For this review, take the finished solid that the model builds, in its own axes (mm). Give positions to 0.01 mm unless a question says otherwise; leave off trailing zeros. Order: outer loops, then holes, each group sorted by start corner. A loop starts at its lowest first (then second) coordinate and runs counter-clockwise, first axis right, second up. Notation, with made-up numbers: M 78,68 L 126,68 A21 cw 126,93 Z; hole C -19.75,10.5 d10. An arc over 180 degrees is marked long. Answer as CSV lines item,"result". Start each with the question number.
1. We need section B-B, the plane x = -94.5. Give the boundary of the cut face in (y, z).
2. For line 1 along X through (y, z) = (7.5, 1.95); line 2 along Y through (x, z) = (106, 0.7), list the stretches that pass through material, from the lowest coordinate up.
3. We need section C-C, the plane z = 1.6. State how many separate pieces and enclosed holes the cut face has, and give its area (3 significant figures).
4. Clearance check with flat-ended pins moving along their axes: P1, Ø1.5, axis at y = -49, z = 2, coming from the -X side; P2, Ø1.5, axis at y = -50, z = 2, coming from the +X side; P3, Ø1.5, axis at x = 43.5, z = 1.5, coming from the -Y side. State where each tip first meets the part, or that it passes through.
5. We need section A-A, the plane y = -37. Give the boundary of the cut face in (x, z).
from build123d import *

# Parameters (mm, degrees)
SKETCH1_W           = 3
SKETCH1_H           = 27
BOSS_EXTRUDE1_DEPTH = 3
SKETCH2_W           = 3
SKETCH2_H           = 27
CUT_EXTRUDE1_DEPTH  = 10
SKETCH3_W           = 27
SKETCH3_H           = 5
BOSS_EXTRUDE3_DEPTH = 3


with BuildPart() as part:
    # Sketch1 → Boss-Extrude1 (new body)
    with BuildSketch(Plane.XY):
        Polygon((-90, 52.5), (-90, 47.5), (-113, 47.5), (-113, 52.5), (-140, 52.5), (-140, 47.5), (-150, 47.5), (-150, -47.5), (150, -47.5), (150, 47.5), (137, 47.5), (137, 52.5), (110, 52.5), (110, 47.5), (87, 47.5), (87, 52.5), (60, 52.5), (60, 47.5), (37, 47.5), (37, 52.5), (10, 52.5), (10, 47.5), (-13, 47.5), (-13, 52.5), (-40, 52.5), (-40, 47.5), (-63, 47.5), (-63, 52.5), align=None)
        with Locations((-147.5, 30.102605219)):
            Rectangle(SKETCH1_W, SKETCH1_H, mode=Mode.SUBTRACT)
        with Locations((-147.5, -29.897394781)):
            Rectangle(SKETCH1_W, SKETCH1_H, mode=Mode.SUBTRACT)
        with Locations((-147.5, 0.102605219)):
            Rectangle(SKETCH1_W, SKETCH1_H, mode=Mode.SUBTRACT)
    extrude(amount=BOSS_EXTRUDE1_DEPTH)

    # Sketch2 → Cut-Extrude1 (cut)
    with BuildSketch(Plane.XY.offset(3)):
        with Locations((141.5, 30.1)):
            Rectangle(SKETCH2_W, SKETCH2_H)
        with Locations((141.5, 0.1)):
            Rectangle(SKETCH2_W, SKETCH2_H)
        with Locations((141.5, -29.9)):
            Rectangle(SKETCH2_W, SKETCH2_H)
    extrude(amount=-CUT_EXTRUDE1_DEPTH, mode=Mode.SUBTRACT)

    # Sketch3 → Boss-Extrude3 (add)
    with BuildSketch(Plane.XY.offset(3)):
        with Locations((-126.5, -50)):
            Rectangle(SKETCH3_W, SKETCH3_H)
        with Locations((-76.5, -50)):
            Rectangle(SKETCH3_W, SKETCH3_H)
        with Locations((-26.5, -50)):
            Rectangle(SKETCH3_W, SKETCH3_H)
        with Locations((23.5, -50)):
            Rectangle(SKETCH3_W, SKETCH3_H)
        with Locations((73.5, -50)):
            Rectangle(SKETCH3_W, SKETCH3_H)
        with Locations((123.5, -50)):
            Rectangle(SKETCH3_W, SKETCH3_H)
    extrude(amount=-BOSS_EXTRUDE3_DEPTH)


solid = part.part
Result set:
1,outline,"M -47.5,0 L 47.5,0 L 47.5,3 L -47.5,3 Z"
2,line 1,"-150 to -149, -146 to 140, 143 to 150"
2,line 2,"-47.5 to 47.5"
3,separate pieces,"1"
3,enclosed holes,"6"
3,area,"29,600 mm2"
4,P1,"x = -140"
4,P2,"x = 137"
4,P3,"y = -47.5"
5,outline,"M -150,0 L -149,0 L -149,3 L -150,3 Z; M -146,0 L 140,0 L 140,3 L -146,3 Z; M 143,0 L 150,0 L 150,3 L 143,3 Z"
